Geometry check sheet. Reference: drawing and pictorial views, mm from the part's lowest x, y, z. Give positions to 0.01 mm unless a question says otherwise; leave off trailing zeros. Loops run counter-clockwise (first coordinate to the right, second up) from the corner with the lowest first, then second, coordinate; pieces in that order, holes last. Notation, with made-up numbers: (-2, -30) - (49, -30) arc R26 cw to (49, 3) - close; hole circle Ø3 at (77, 32). An arc over 180 degrees is marked (long way). Answer in a Markdown table with one row per item. Add a question column.
(1) Go/stop test with a flat-tipped pin: P1, Ø0.9, axis at x = 4, y = 21, coming from the +Z side. Record where the tip stops, or that it passes through.
(2) Sectioned sample at A-A on z = 9. Enter the section's corners in (x, y).
(3) Thickness scan on L1, parallel to Y at x = 4, z = 17; L2, parallel to Y at x = 24, z = 20.25; L3, parallel to Z at x = 25.75, y = 8.75. Record the ranges inside material, lowest first.
(4) Draft check along X on the marked faces 1, 2 and 3. Enter one of: released by +X, released by -X, zero draft, split by the parting line, or undercut.
(5) Sectioned sample at D-D on x = 4. Enter the section's corners in (y, z).
(6) Sectioned sample at C-C on y = 17.75. Enter the section's corners in (x, z).
(7) Sectioned sample at B-B on x = 18.1. Enter the section's corners in (y, z), then the cut area to 4 significant figures.
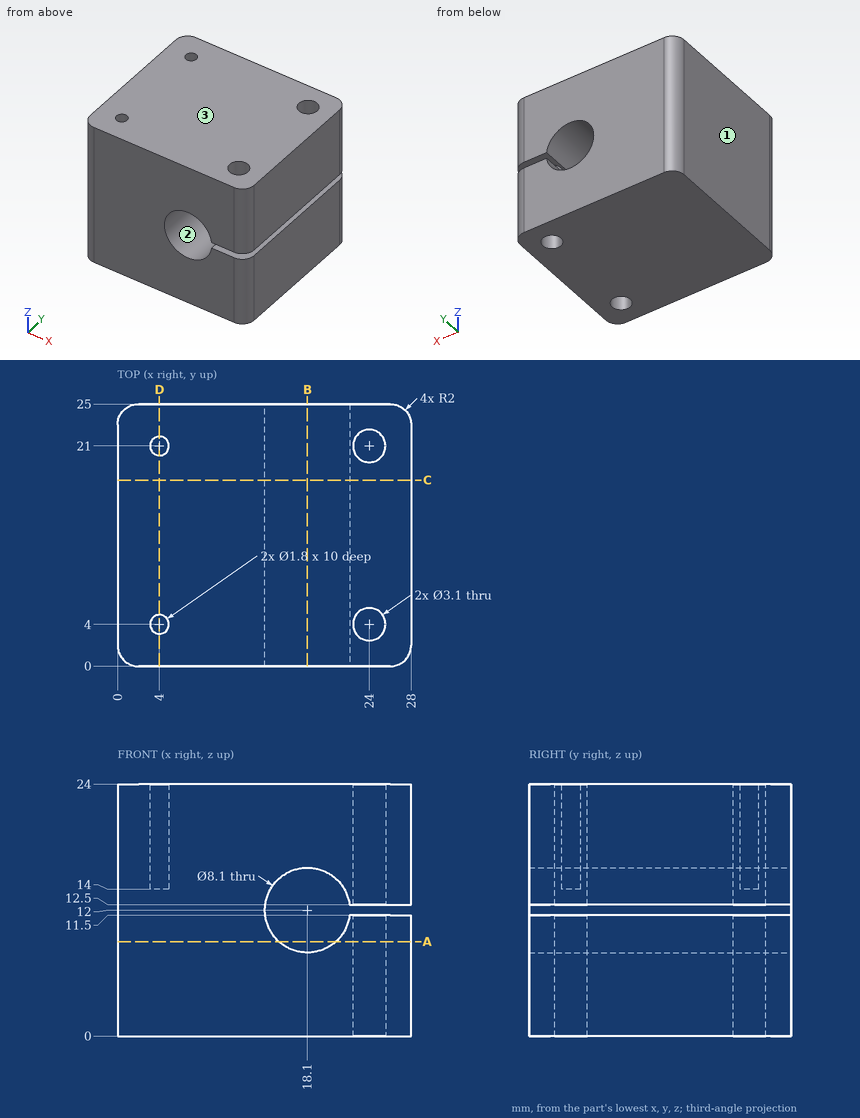
Reply:
| question | item | result |
|---|---|---|
| 1 | P1 | z = 14 |
| 2 | outline | (0, 2) arc R2 ccw to (2, 0) - (15.38, 0) - (15.38, 25) - (2, 25) arc R2 ccw to (0, 23) - close; (20.82, 0) - (26, 0) arc R2 ccw to (28, 2) - (28, 23) arc R2 ccw to (26, 25) - (20.82, 25) - close; hole circle Ø3.1 at (24, 4); hole circle Ø3.1 at (24, 21) |
| 3 | L1 | 0 to 3.1, 4.9 to 20.1, 21.9 to 25 |
| 3 | L2 | 0 to 2.45, 5.55 to 19.45, 22.55 to 25 |
| 3 | L3 | 0 to 11.5, 12.5 to 24 |
| 4 | face 1 | released by -X |
| 4 | face 2 | undercut |
| 4 | face 3 | zero draft |
| 5 | outline | (0, 0) - (25, 0) - (25, 24) - (21.9, 24) - (21.9, 14) - (20.1, 14) - (20.1, 24) - (4.9, 24) - (4.9, 14) - (3.1, 14) - (3.1, 24) - (0, 24) - close |
| 6 | outline | (0, 0) - (28, 0) - (28, 11.5) - (22.12, 11.5) arc R4.05 cw (long way) to (22.12, 12.5) - (28, 12.5) - (28, 24) - (0, 24) - close |
| 7 | outline | (0, 0) - (25, 0) - (25, 7.95) - (0, 7.95) - close; (0, 16.05) - (25, 16.05) - (25, 24) - (0, 24) - close |
| 7 | area | 397.5 mm^2 |
